Autodesk Inventor part; units mm, degrees
ref_plane "Work Plane1" through (-20.2583, -25.7942, 0) normal (0, 0, 1) x (1, 0, 0)
ref_plane "Work Plane4" through (8.9999, -18.0001, 0) normal (1, 0, 0) x (0, 0, -1)
ref_plane "YZ Plane" through (0, 0, 0) normal (1, 0, 0) x (0, 1, 0)
sketch "Sketch1" plane through (0, 0, 0) normal (0, 0, 1) x (1, 0, 0)
  circle A0 centre (-0.0001, 55.0001) radius 2.5
  line L0 (-9, 60.0001) -> (-9, 34.0001)
  line L1 (-9, 34.0001) -> (-5.0001, 34.0001)
  line L2 (-5.0001, 34.0001) -> (-5.0001, 45.0001)
  line L3 (-5.0001, 45.0001) -> (4.9999, 45.0001)
  line L4 (4.9999, 45.0001) -> (4.9999, 34.0001)
  line L5 (4.9999, 34.0001) -> (8.9999, 34.0001)
  line L6 (8.9999, 34.0001) -> (8.9999, 60.0001)
  line L7 (8.9999, 60.0001) -> (-9, 60.0001)
  line L8 (-9, 8) -> (-9, -18)
  line L9 (-5, -18) -> (-5, -8)
  circle A1 centre (-0.0001, -13.0001) radius 2.5
  line L10 (8.9999, -18.0001) -> (8.9999, 7.9999)
  line L11 (8.9999, 7.9999) -> (4.9999, 7.9999)
  line L12 (4.9999, 7.9999) -> (4.9999, 2.5001)
  line L13 (5, -3) -> (-5.0001, -3.0001)
  line L14 (-5.0001, -3.0001) -> (-5.0001, 7.9999)
  line L15 (-5.0001, 7.9999) -> (-9, 7.9999)
  line L16 (-9, -18.0001) -> (8.9999, -18.0001)
  line L17 (8.9999, 60.0001) -> (-9, 60.0001)
  line L18 (-9, 60.0001) -> (-9, -18)
  line L19 (-9, -18) -> (8.9999, -18)
  line L20 (8.9999, -18) -> (8.9999, 60.0001)
  circle A2 centre (-0.0001, 55.0001) radius 2.5
  circle A3 centre (-0.0001, -13.0001) radius 2.5
  line L21 (-9, 7.9999) -> (-9, -18.0001)
  line L22 (4.9999, 2.5001) -> (5, -3)
  point P0 (0, 0)
  dimension "d0" = 4
  dimension "d1" = 0
extrude "Extrusion1" add sketch "Sketch1" along normal blind 4
sketch "Sketch2" plane through (0, 0, 4) normal (0, 0, 1) x (1, 0, 0)
  circle A0 centre (-55.3, -73.0192) radius 2.5
  circle A1 centre (-55.3001, 115.0193) radius 2.5
  line L0 (-55.3, -73.0192) -> (33.584, 75.4143)
  line L1 (-55.3001, 115.0193) -> (26.1085, -20.9304)
  line L2 (-9, 60) -> (-9, -18)
  line L3 (-9, 21) -> (62.9573, 21)
  line L4 (1, 21) -> (-7.5794, 15.8625)
  line L5 (-55.3001, 115.0193) -> (-50.1626, 106.4399)
  line L6 (-50.1626, 106.4399) -> (-41.5832, 111.5774)
  line L7 (-50.1626, 106.4399) -> (-58.742, 101.3024)
  line L8 (-7.5794, 15.8625) -> (-58.742, 101.3024)
  line L9 (1, 21) -> (9.5794, 26.1375)
  line L10 (9.5794, 26.1375) -> (-41.5832, 111.5774)
  line L11 (1, 21) -> (-7.5794, 26.1375)
  line L12 (1, 21) -> (9.5794, 15.8625)
  line L13 (-55.3, -73.0192) -> (-50.1625, -64.4398)
  line L14 (-93.1275, -68.5) -> (-47.8, -94.6699)
  line L15 (-50.1625, -64.4398) -> (-41.5831, -69.5773)
  line L16 (-50.1625, -64.4398) -> (-58.742, -59.3023)
  line L17 (-41.5831, -69.5773) -> (9.5794, 15.8625)
  line L18 (-7.5794, 26.1375) -> (-58.742, -59.3023)
  line L19 (-10.6558, 21) -> (6.503, 31.2749)
  line L20 (-10.6558, 21) -> (6.503, 10.7251)
  circle A2 centre (-0.0001, -13.0001) radius 2.5
  circle A3 centre (-0.0001, -13.0001) radius 5
  circle A4 centre (-0.0001, 55.0001) radius 2.5
  circle A5 centre (-0.0001, 55.0001) radius 5
  line L21 (8.9999, 60.0001) -> (-9, 60.0001)
  line L22 (-9, -18.0001) -> (8.9999, -18.0001)
  line L23 (-20.2607, 4.9602) -> (12.7451, -14.8042)
  line L24 (-20.2607, 37.0398) -> (12.7451, 56.8042)
  line L25 (-20.2607, 4.9602) -> (-22.8345, 6.5014)
  line L26 (-9, 21) -> (-33.1607, 21)
  line L27 (-22.8345, 6.5014) -> (-14.1525, 21)
  line L28 (-20.2607, 37.0398) -> (-22.8345, 35.4986)
  line L29 (-22.8345, 35.4986) -> (-14.1525, 21)
  line L30 (6.503, 10.7251) -> (8.9999, 9.2299)
  line L31 (8.9999, -18.0001) -> (8.9999, 60.0001)
  line L32 (6.503, 31.2749) -> (8.9999, 32.7701)
  line L33 (8.9999, 32.7701) -> (-0.605, 48.8099)
  line L34 (8.9999, 9.2299) -> (-0.605, -6.8099)
  line L35 (8.9999, 32.7701) -> (8.9999, 9.2299)
  line L36 (-22.8345, 6.5014) -> (-22.8345, 35.4986)
  point P0 (0, 0)
  point P1 (-20.2607, 37.0398)
  point P2 (6.503, 10.7251)
  point P3 (-3.1018, -5.3148)
  point P4 (8.524, 8.4352)
  point P5 (7.516, 10.1185)
  point P6 (-3.1019, 47.3148)
  point P7 (6.503, 31.2749)
  point P8 (-2.0764, 26.1375)
  point P9 (-11.6813, 42.1773)
  point P10 (6.8279, 11.2676)
  point P11 (8.9999, 14.8947)
  point P12 (8.9999, 16.2096)
  point P13 (6.503, 10.7251)
  point P14 (8.9999, 25.7904)
  point P15 (6.503, 31.2749)
  point P16 (8.9999, 27.1053)
  point P17 (8.9999, 32.7701)
  point P18 (8.9999, 32.7704)
  point P19 (8.9999, 9.2299)
  point P20 (8.9999, 7.6404)
  point P21 (8.9999, 9.2296)
  point P22 (8.9999, 54.5615)
  point P23 (8.9999, -12.5615)
  dimension "d0" = 4
  dimension "d1" = 0
  dimension "d2" = 10
  dimension "d3" = 10
  dimension "d4" = 10
  dimension "d5" = 10
  dimension "d6" = 10
  dimension "d7" = 10
  dimension "d8" = 10
  dimension "d9" = 10
  dimension "d10" = 10
  dimension "d11" = 10
  dimension "d12" = 10
  dimension "d13" = 20
  dimension "d14" = 20
  dimension "d15" = 3
  dimension "d16" = 3
extrude "Extrusion2" add sketch "Sketch2" along normal blind 20 contours L25 L27 L26 L18 | L20 L4 L0 | L0 L1 L17 L20 | L26 L29 L28 L8 | L26 L2 L20 | L19 L2 L26 | L17 L30 L1 L34 L23 | L1 L19 L10 L0 | L11 L19 L1 | L12 L31 L17 L1 | L4 L20 L2 L3 | L9 L31 L3 | L0 L10 L31 L9 | L3 L2 L19 L11 | L3 L31 L12 | L17 L1 L30 | L34 L1 L31 L23 | L10 L32 L0 | L0 L32 L31 L10 | L17 L31 L30 L1 | L30 L34 L1 | L34 L31 L1 | L32 L10 L24 L33 L0 | L0 L33 L32 | L33 L24 L31 L0 | L0 L31 L33
sketch "Sketch3" plane through (0, 0, 4) normal (0, 0, -1) x (-1, 0, 0)
  line L0 (10.6558, 21) -> (20.2607, 37.0398)
  line L1 (20.2607, 37.0398) -> (8.9915, 37.0398)
  line L2 (20.2607, 4.9602) -> (10.6558, 21)
  line L3 (20.2607, 4.9602) -> (9, 4.9602)
  line L4 (9, 20.0085) -> (9, -18)
  line L5 (22.8345, 35.4986) -> (14.1525, 21)
  line L6 (22.8345, 6.5014) -> (20.2607, 4.9602)
  line L7 (22.8345, 35.4986) -> (22.8345, 6.5014)
  line L8 (9, 60) -> (9, -18)
  line L9 (10.6558, 21) -> (9, 20.0085)
  line L10 (9, 21.9915) -> (10.6558, 21)
  line L11 (22.8345, 6.5014) -> (20.2607, 4.9602)
  line L12 (14.1525, 21) -> (22.8345, 6.5014)
  line L13 (22.8345, 35.4986) -> (14.1525, 21)
  line L14 (20.2607, 37.0398) -> (22.8345, 35.4986)
  line L15 (10.6558, 21) -> (20.2607, 37.0398)
  line L16 (20.2607, 4.9602) -> (10.6558, 21)
  line L17 (-8.9999, 60.0001) -> (9, 60.0001)
  line L18 (-8.9999, -18.0001) -> (-8.9999, 60.0001)
  line L19 (9, -18.0001) -> (-8.9999, -18.0001)
  circle A0 centre (0.0001, -13.0001) radius 2.5
  circle A1 centre (0.0001, 55.0001) radius 2.5
  line L20 (9, 60.0001) -> (9, -18.0001)
  point P0 (0, 0)
  point P1 (9, 37.0398)
  dimension "d0" = 4
  dimension "d1" = 0
ref_plane "Work Plane1" through (-20.2583, -25.7942, 0) normal (0, 0, 1) x (1, 0, 0)
extrude "Extrusion3" add sketch "Sketch3" along normal up to surface (4 mm away) contours L10 L8 L1 L0 | L0 L14 L5 L12 L6 L2 | L2 L3 L4 L9 | L9 L8 L10 | L7 L12 L5
ref_plane "Work Plane4" through (8.9999, -18.0001, 0) normal (1, 0, 0) x (0, 0, -1)
sketch "Sketch12" plane through (0, 0, 24) normal (0, 0, 1) x (1, 0, 0)
  line L0 (-3.1018, -5.3148) -> (8.9999, -12.5615)
  line L1 (-14.1525, 21) -> (-22.8345, 6.5014)
  line L2 (8.9999, -12.5615) -> (-22.8345, 6.5014)
  line L3 (-22.8345, 6.5014) -> (-14.1525, 21)
  line L4 (-22.8345, 35.4986) -> (-14.1525, 21)
  line L5 (-14.1525, 21) -> (-22.8345, 35.4986)
  line L6 (-22.8345, 35.4986) -> (8.9999, 54.5615)
  line L7 (8.9999, 54.5615) -> (8.9999, -12.5615)
  point P0 (0, 0)
extrude "Extrusion12" add sketch "Sketch12" along normal blind 3
sketch "Sketch13" plane through (0, 0, 27) normal (0, 0, 1) x (1, 0, 0)
  line L0 (8.9999, -12.5615) -> (8.9999, 54.5615)
  line L1 (8.9999, 21) -> (14.9999, 21)
  line L2 (8.9999, 21) -> (8.9999, 6)
  line L3 (8.9999, 21) -> (8.9999, 36)
  arc A0 (8.9999, 6) -> (8.9999, 36) centre (-6.7501, 21) ccw
  point P0 (0, 0)
  dimension "d52" = 6
  dimension "d53" = 15
  dimension "d54" = 15
extrude "Extrusion13" add sketch "Sketch13" against normal up to surface (27 mm away)
sketch "Sketch14" plane through (0, 0, 27) normal (0, 0, 1) x (1, 0, 0)
  arc A0 (8.9999, 6) -> (8.9999, 36) centre (-6.7501, 21) ccw
  line L0 (14.9999, 21) -> (7.9999, 21)
  circle A1 centre (7.9999, 21) radius 2.5
  point P0 (0, 0)
  dimension "d57" = 7
  dimension "d58" = 5
extrude "Extrusion14" cut sketch "Sketch14" against normal up to surface (23 mm away)
sketch "Sketch15" plane through (8.9999, -18.0001, 4) normal (1, 0, 0) x (0, 0, -1)
  line L0 (-23, 54.0001) -> (-23, 24.0001)
  line L1 (-23, 39.0001) -> (-10, 39.0001)
  line L2 (0, 39.0001) -> (-20, 39.0001)
  line L3 (-17.5, 31.5001) -> (-2.5, 31.5001)
  line L4 (-2.5, 31.5001) -> (-2.5, 46.5001)
  line L5 (-2.5, 46.5001) -> (-17.5, 46.5001)
  line L6 (-17.5, 46.5001) -> (-17.5, 31.5001)
  line L7 (-17.5, 31.5001) -> (-2.5, 46.5001) construction
  line L8 (-2.5, 31.5001) -> (-17.5, 46.5001) construction
  point P0 (4, 18.0001)
  dimension "d61" = 15
  dimension "d62" = 15
extrude "Extrusion15" cut sketch "Sketch15" along normal blind 10 and the other way blind 7
sketch "Sketch16" plane through (0, 0, 27) normal (0, 0, 1) x (1, 0, 0)
  line L0 (-3.1018, -5.3148) -> (6.503, 10.7251)
  line L1 (6.503, 31.2749) -> (-3.1019, 47.3148)
  line L2 (-3.1018, -5.3148) -> (-1.386, -6.3423)
  line L3 (-22.8345, 6.5014) -> (8.9999, -12.5615)
  line L4 (-1.386, -6.3423) -> (4.4507, 3.4048)
  line L5 (8.9999, -12.5615) -> (8.9999, 6)
  line L6 (8.9999, 6) -> (-9.8503, 6)
  line L7 (4.4507, 3.4048) -> (6.0048, 6)
  line L8 (-22.8345, 35.4986) -> (-14.1525, 21)
  line L9 (-14.1525, 21) -> (17.1457, 21)
  line L10 (-22.8345, 35.4986) -> (8.9999, 54.5615)
  line L11 (-1.386, 48.3423) -> (4.4507, 38.5952)
  line L12 (8.9999, 54.5615) -> (8.9999, 36)
  line L13 (8.9999, 36) -> (-9.8503, 36)
  line L14 (4.4507, 38.5952) -> (6.0048, 36)
  point P0 (0, 0)
  dimension "d67" = 2
extrude "Extrusion16" cut sketch "Sketch16" against normal up to surface (23 mm away) contours L4 L7 L6 L5 L3 | L14 L11 L10 L12 L13
sketch "Sketch17" plane through (6.0048, 6, 27) normal (0.8579416, -0.5137472, 0) x (0, 0, -1)
  line L0 (0, 2.5134) -> (0, -14.3859)
  line L1 (0, -8.2326) -> (13, -8.2326)
  circle A0 centre (13, -8.2326) radius 1.5
  point P0 (27, -8.2326)
  dimension "d71" = 13
  dimension "d72" = 3
extrude "Extrusion17" cut sketch "Sketch17" against normal through all
sketch "Sketch18" plane through (6.0048, 36, 27) normal (0.8579416, 0.5137472, 0) x (0, 0, -1)
  line L0 (23, 14.3859) -> (0, 14.3859)
  line L1 (0, 14.3859) -> (0, 8.2329)
  line L2 (0, 14.3859) -> (0, -2.5134)
  line L3 (0, 8.2329) -> (13, 8.2329)
  circle A0 centre (13, 8.2329) radius 1.5
  point P0 (27, -27.801)
  dimension "d75" = 6.153
  dimension "d76" = 13
  dimension "d77" = 3
extrude "Extrusion18" cut sketch "Sketch18" against normal through all
properties part number "2020_top_guide_mnt" material "PET Plastic"
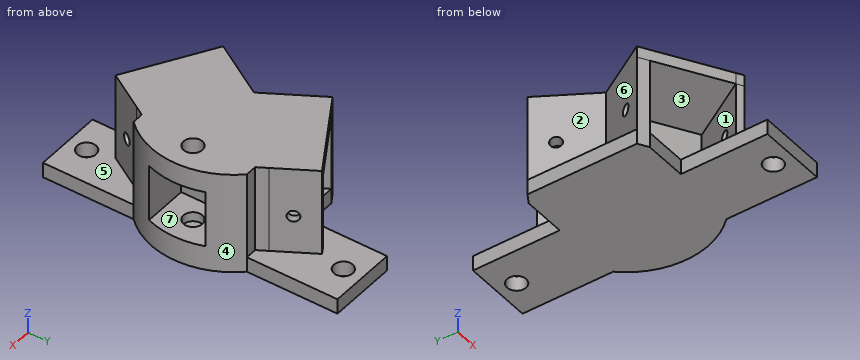
The listing builds one solid part. Answer for the finished solid, in the listing's coordinates (mm). Face numbers are marked on the shaded views. A direction names the side the tool comes from. Coordinates: 2 decimals unless noted, no trailing zeros. Write each loop counter-clockwise with the first axis right and the second up, starting at its lowest first coordinate (ties: lowest second). Pieces come first, ordered by that corner, then holes. Notation, with made-up numbers: M -11.5,25 L 14.5,25 A5 ccw 14.5,29 Z; hole C -18.5,43.5 d8. An arc over 180 degrees is marked long. Put each result on its own line as item: value. Start each with the question number.
1. Flat-ended cylindrical pins translate along their axes: P1, Ø5, axis at x = 8, z = 23, coming from the +Y side; P2, Ø2, axis at y = 41, z = 8, coming from the +X side; P3, Ø4.5, axis at x = -14, z = 1.5, coming from the +Y side; P4, Ø1.5, axis at x = 11, y = 44, coming from the +Z side. Find the tip coordinate at first contact, or state that the pin passes through.
2. Consider line 1 (Y direction, x = 7, z = 21); line 2 (Z direction, x = 6.5, y = 18.5); line 3 (Z direction, x = -6, y = 11). Determine where each line is inside the solid, lowest interval first. Write a range as from..to.
3. Which of the six approach directions +Z, -Z, +X, -X, +Y, -Y give full straight-line access (tool end or side, diameter ignored) to the marked faces 5, 6 and 7?
4. A cutting plane is placed at B-B on y = 27.5. Write down the section's boundary in (x, z).
5. For a pull along X with two mould halves and no side action, classify the marked faces 1, 2, 3 and 4 as pulls with the +X half, pulls with the -X half, needs draft (parallel to the pull), parting line crosses it, or undercut.
Resolved:
1. P1: stops at y = 36.84
1. P2: stops at x = 3.61
1. P3: stops at y = 37.04
1. P4: passes through
2. line 1: y = 6..13.5, 28.5..36
2. line 2: z = 0..6.5, 21.5..27
2. line 3: z = 0..4, 24..27
3. face 5: none
3. face 6: +Z, -X
3. face 7: +X
4. outline: M -22.83,0 L 14.01,0 L 14.01,6.5 L 2,6.5 L 2,21.5 L 14.01,21.5 L 14.01,27 L -18.04,27 L -18.04,4 L -22.83,4 Z; hole M -14.55,4 L 0.2,4 L 0.2,24 L -14.55,24 Z
5. face 1: undercut
5. face 2: pulls with the -X half
5. face 3: undercut
5. face 4: pulls with the +X half
